```python
from build123d import *

# Parameters (mm, degrees)
F0_W     = 74.4
F0_H     = 39.6
F0_R     = 1
F0_R_2   = 4.1
F1_DEPTH = 1.5
F2_W     = 30
F2_H     = 1.5
F3_DEPTH = 44
F4_R     = 1.1
F4_R_2   = 4.1
F5_DEPTH = 1.5
F6_R     = 5
F7_W     = 74.4
F7_H     = 39.6
F8_DEPTH = 1.5
F9_R     = 5


with BuildPart() as f1:
    # F0 (on Top) → F1 (new body)
    with BuildSketch(Plane.XY):
        Rectangle(F0_W, F0_H)
        with Locations((-32.2, -16.8)):
            Circle(F0_R, mode=Mode.SUBTRACT)
        with Locations((-25, -10.6)):
            Circle(F0_R_2, mode=Mode.SUBTRACT)
        with Locations((-17.8, -16.8)):
            Circle(F0_R, mode=Mode.SUBTRACT)
        with Locations((17.8, -16.8)):
            Circle(F0_R, mode=Mode.SUBTRACT)
        with Locations((32.2, -16.8)):
            Circle(F0_R, mode=Mode.SUBTRACT)
        with Locations((25, -10.6)):
            Circle(F0_R_2, mode=Mode.SUBTRACT)
        with BuildLine():
            ThreePointArc((-34.8, 11.6), (-34.507107, 12.307107), (-33.8, 12.6))
            Line((-33.8, 12.6), (-30.123475, 12.6))
            ThreePointArc((-30.123475, 12.6), (-25, 15.1), (-19.876525, 12.6))
            Line((-19.876525, 12.6), (-16.2, 12.6))
            ThreePointArc((-16.2, 12.6), (-15.492893, 12.307107), (-15.2, 11.6))
            Line((-15.2, 11.6), (-15.2, 1.9))
            ThreePointArc((-15.2, 1.9), (-16.664466, -1.635534), (-20.2, -3.1))
            Line((-20.2, -3.1), (-29.8, -3.1))
            ThreePointArc((-29.8, -3.1), (-33.335534, -1.635534), (-34.8, 1.9))
            Line((-34.8, 1.9), (-34.8, 11.6))
        make_face(mode=Mode.SUBTRACT)
        with Locations((-32.2, 14.8)):
            Circle(F0_R, mode=Mode.SUBTRACT)
        with Locations((-17.8, 14.8)):
            Circle(F0_R, mode=Mode.SUBTRACT)
        with BuildLine():
            Line((15.2, 1.9), (15.2, 11.6))
            ThreePointArc((15.2, 11.6), (15.492893, 12.307107), (16.2, 12.6))
            Line((16.2, 12.6), (19.876525, 12.6))
            ThreePointArc((19.876525, 12.6), (25, 15.1), (30.123475, 12.6))
            Line((30.123475, 12.6), (33.8, 12.6))
            ThreePointArc((33.8, 12.6), (34.507107, 12.307107), (34.8, 11.6))
            Line((34.8, 11.6), (34.8, 1.9))
            ThreePointArc((34.8, 1.9), (33.335534, -1.635534), (29.8, -3.1))
            Line((29.8, -3.1), (20.2, -3.1))
            ThreePointArc((20.2, -3.1), (16.664466, -1.635534), (15.2, 1.9))
        make_face(mode=Mode.SUBTRACT)
        with Locations((17.8, 14.8)):
            Circle(F0_R, mode=Mode.SUBTRACT)
        with Locations((32.2, 14.8)):
            Circle(F0_R, mode=Mode.SUBTRACT)
    extrude(amount=F1_DEPTH)

    # F2 (on Top) → F3 (join)
    with BuildSketch(Plane.XY):
        with Locations((0, 20.55)):
            Rectangle(F2_W, F2_H)
    extrude(amount=F3_DEPTH)

    # F4 (on face) → F5 (cut, through all)
    with BuildSketch(Plane(origin=(0, 21.3, 0), x_dir=(-1, 0, 0), z_dir=(0, 1, 0))):
        with Locations((7.2, 41)):
            Circle(F4_R)
        with Locations((7.2, 9.9)):
            Circle(F4_R)
        with Locations((0, 16.1)):
            Circle(F4_R_2)
        with BuildLine():
            ThreePointArc((9.8, 37.9), (9.507107, 38.607107), (8.8, 38.9))
            Line((8.8, 38.9), (5.499091, 38.9))
            ThreePointArc((5.499091, 38.9), (5.099091, 38.983485), (4.765879, 39.22))
            ThreePointArc((4.765879, 39.22), (0, 41.3), (-4.765879, 39.22))
            ThreePointArc((-4.765879, 39.22), (-5.099091, 38.983485), (-5.499091, 38.9))
            Line((-5.499091, 38.9), (-8.8, 38.9))
            ThreePointArc((-8.8, 38.9), (-9.507107, 38.607107), (-9.8, 37.9))
            Line((-9.8, 37.9), (-9.8, 28.2))
            ThreePointArc((-9.8, 28.2), (-8.335534, 24.664466), (-4.8, 23.2))
            Line((-4.8, 23.2), (4.8, 23.2))
            ThreePointArc((4.8, 23.2), (8.335534, 24.664466), (9.8, 28.2))
            Line((9.8, 28.2), (9.8, 37.9))
        make_face()
        with Locations((-7.2, 41)):
            Circle(F4_R)
        with Locations((-7.2, 9.9)):
            Circle(F4_R)
    extrude(amount=-F5_DEPTH, mode=Mode.SUBTRACT)

    # F6
    f6_edges = [f1.edges().sort_by_distance(p)[0] for p in [
        (-37.2, 19.8, 0.75),
        (-37.2, -19.8, 0.75),
        (37.2, 19.8, 0.75),
        (37.2, -19.8, 0.75),
        (-15, 20.55, 44),
        (15, 20.55, 44),
    ]]
    fillet(f6_edges, radius=F6_R)

    # F7 (on face) → F8 (cut, through all)
    with BuildSketch(Plane.XY.offset(1.5)):
        Rectangle(F7_W, F7_H)
    extrude(amount=-F8_DEPTH, mode=Mode.SUBTRACT)

    # F9
    f9_edges = [f1.edges().sort_by_distance(p)[0] for p in [
        (-15, 20.55, 0),
        (15, 20.55, 0),
    ]]
    fillet(f9_edges, radius=F9_R)


solid = f1.part
```
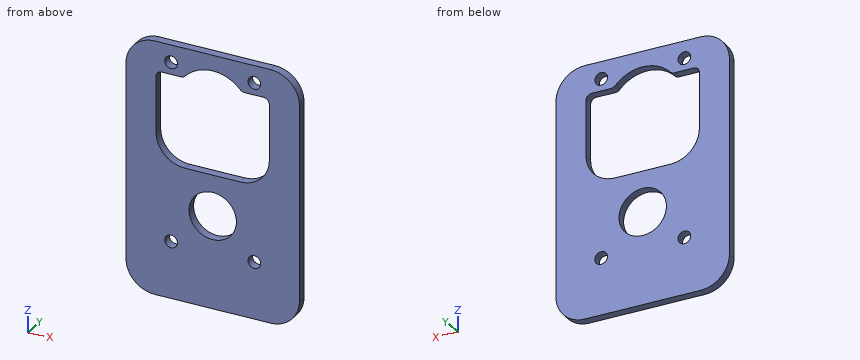
Geometry check sheet. Reference: the model listing, model coordinates, mm. Round coordinates to 2 decimals unless told otherwise and drop trailing zeros. Loops run counter-clockwise (first coordinate to the right, second up) from the corner with the lowest first, then second, coordinate; pieces in that order, holes last. Notation, with made-up numbers: M 77,-26 L 96,-26 A22 ccw 96,10 Z; hole C 79.25,5 d9. An arc over 180 degrees is marked long. Return JSON: item names as keys, results as strings. Group by question number.
(1) Scan lines: line 1 along Z through (x, y) = (0, 20.45); line 2 along X through (y, z) = (20.9, 38); line 3 along Z through (x, y) = (7.2, 20.2). Record each from-to range of solid material in increasing order. Write a range as [from, to].
(2) Section check C-C, the plane y = 20.25. Enter the section's corners in (x, z).
(3) Section check B-B, the plane x = 0. Enter the section's corners in (y, z).
(4) Section check A-A, the plane z = 31. Enter the section's corners in (x, y).
(5) Section check D-D, the plane x = -7.2. Enter the section's corners in (y, z), and give its area (3 significant figures).
Data:
{
 "1": {"line 1": "[0, 12], [20.2, 23.2], [41.3, 44]", "line 2": "[-15, -9.79], [9.79, 15]", "line 3": "[0, 8.8], [11, 23.81], [38.9, 39.9], [42.1, 44]"},
 "2": {"outline": "M -15,5 A5 ccw -10,0 L 10,0 A5 ccw 15,5 L 15,39 A5 ccw 10,44 L -10,44 A5 ccw -15,39 Z; hole M -9.8,28.2 A5 ccw -4.8,23.2 L 4.8,23.2 A5 ccw 9.8,28.2 L 9.8,37.9 A1 ccw 8.8,38.9 L 5.5,38.9 A1 cw 4.77,39.22 A6.5 ccw -4.77,39.22 A1 cw -5.5,38.9 L -8.8,38.9 A1 ccw -9.8,37.9 Z; hole C -7.2,9.9 d2.2; hole C -7.2,41 d2.2; hole C 0,16.1 d8.2; hole C 7.2,9.9 d2.2; hole C 7.2,41 d2.2"},
 "3": {"outline": "M 19.8,0 L 21.3,0 L 21.3,12 L 19.8,12 Z; M 19.8,20.2 L 21.3,20.2 L 21.3,23.2 L 19.8,23.2 Z; M 19.8,41.3 L 21.3,41.3 L 21.3,44 L 19.8,44 Z"},
 "4": {"outline": "M -15,19.8 L -9.8,19.8 L -9.8,21.3 L -15,21.3 Z; M 9.8,19.8 L 15,19.8 L 15,21.3 L 9.8,21.3 Z"},
 "5": {"outline": "M 19.8,0 L 21.3,0 L 21.3,8.8 L 19.8,8.8 Z; M 19.8,11 L 21.3,11 L 21.3,23.81 L 19.8,23.81 Z; M 19.8,38.9 L 21.3,38.9 L 21.3,39.9 L 19.8,39.9 Z; M 19.8,42.1 L 21.3,42.1 L 21.3,44 L 19.8,44 Z", "area": "36.8 mm²"}
}
